from build123d import *

# Parameters (mm, degrees)
BOSS_EXTRUDE1_DEPTH = 6.35
FILLET1_R           = 6.35
SKETCH2_R           = 3.175
CUT_EXTRUDE1_DEPTH  = 6.35
BOSS_EXTRUDE2_START = 0.396875
SKETCH3_R           = 6.35
SKETCH3_R_2         = 3.175
BOSS_EXTRUDE2_DEPTH = 0.396875
SKETCH4_R           = 6.35
SKETCH4_R_2         = 3.175
BOSS_EXTRUDE3_DEPTH = 0.396875
FILLET2_R           = 1.5875
CHAMFER1_SIZE       = 3.175
FILLET3_R           = 3.175


with BuildPart() as part:
    # Sketch1 → Boss-Extrude1 (new body)
    with BuildSketch(Plane.XY):
        Polygon((0, 0), (38.1, 0), (42.964382214, -4.081701322), (59.2911875, 15.375827534), (47.023929506, 18.662829407), (35.810782514, 12.7), (0, 12.7), align=None)
    extrude(amount=BOSS_EXTRUDE1_DEPTH)

    # Fillet1
    fillet1_edges = [part.edges().sort_by_distance(p)[0] for p in [
        (47.023929506, 18.662829407, 3.175),
        (0, 0, 3.175),
        (0, 12.7, 3.175),
    ]]
    fillet(fillet1_edges, radius=FILLET1_R - 0.0001)  # a hair under: the kernel refuses the full size

    # Sketch2 → Cut-Extrude1 (cut)
    with BuildSketch(Plane.XY.offset(6.35)):
        with Locations((6.35, 6.35)):
            Circle(SKETCH2_R)
        with Locations((31.75, 6.35)):
            Circle(SKETCH2_R)
    extrude(amount=-CUT_EXTRUDE1_DEPTH, mode=Mode.SUBTRACT)

    # Sketch3 → Boss-Extrude2 (add)
    # profile 1 of 2: a face of its own
    with BuildSketch(Plane.XY.offset(6.35).offset(BOSS_EXTRUDE2_START)):
        with Locations(Location((31.75, 6.35, 0), (0, 0, 270))):
            Circle(SKETCH3_R)
        with Locations((31.75, 6.35)):
            Circle(SKETCH3_R_2, mode=Mode.SUBTRACT)
    # profile 2 of 2: a face of its own
    with BuildSketch(Plane.XY.offset(6.35).offset(BOSS_EXTRUDE2_START)):
        with Locations(Location((6.35, 6.35, 0), (0, 0, 180))):
            Circle(SKETCH3_R)
        with Locations((6.35, 6.35)):
            Circle(SKETCH3_R_2, mode=Mode.SUBTRACT)
    extrude(amount=-BOSS_EXTRUDE2_DEPTH)

    # Sketch4 → Boss-Extrude3 (add)
    # profile 1 of 2: a face of its own
    with BuildSketch(Plane(origin=(0, 0, 0), x_dir=(-1, 0, 0), z_dir=(0, 0, -1))):
        with Locations(Location((-31.75, 6.35, 0), (0, 0, 270))):
            Circle(SKETCH4_R)
        with Locations(Location((-31.75, 6.35, 0), (0, 0, 180))):
            Circle(SKETCH4_R_2, mode=Mode.SUBTRACT)
    # profile 2 of 2: a face of its own
    with BuildSketch(Plane(origin=(0, 0, 0), x_dir=(-1, 0, 0), z_dir=(0, 0, -1))):
        with Locations((-6.35, 6.35)):
            Circle(SKETCH4_R)
        with Locations(Location((-6.35, 6.35, 0), (0, 0, 180))):
            Circle(SKETCH4_R_2, mode=Mode.SUBTRACT)
    extrude(amount=BOSS_EXTRUDE3_DEPTH)

    # Fillet2
    fillet2_edges = [part.edges().sort_by_distance(p)[0] for p in [
        (59.2911875, 15.375827534, 3.175),
        (38.1, 0, 3.175),
    ]]
    fillet(fillet2_edges, radius=FILLET2_R)

    # Chamfer1
    chamfer1_edges = [part.edges().sort_by_distance(p)[0] for p in [
        (42.964382214, -4.081701322, 3.175),
    ]]
    chamfer(chamfer1_edges, length=CHAMFER1_SIZE)

    # Fillet3
    fillet3_edges = [part.edges().sort_by_distance(p)[0] for p in [
        (45.005232875, -1.649510215, 3.175),
        (40.532191107, -2.040850661, 3.175),
    ]]
    fillet(fillet3_edges, radius=FILLET3_R)


solid = part.part
Design review of the part built by this model. Coordinates are the model's own, in mm. A direction names the side the tool comes from. Coordinates: 2 decimals unless noted, no trailing zeros. Write each loop counter-clockwise with the first axis right and the second up, starting at its lowest first coordinate (ties: lowest second). Pieces come first, ordered by that corner, then holes. Notation, with made-up numbers: (83.5, 48.5) -> (92.5, 48.5) arc R23 cw to (92.5, 67.5) -> close; hole circle Ø2 at (21.25, 62). An arc over 180 degrees is marked (long way). Write each question's results on one line, items separated by ' | '. Start each with the question number.
(1) Take a section at B-B on x = 4.5. Write out the cut boundary in (y, z).
(2) Tool access review of faces 4 (the face through (21, 12.7, 3)), 5 (the face through (44.9, -1.41, 3.22)), 6 (the face through (33.657, 0.293, 6.551)): name each direction out of +Z, -Z, +X, -X, +Y, -Y from which nothing blocks a thin tool from reaching the whole face with its end or side.
(3) The part is to be moulded in two halves that separate along Y. For faces 1 (the face through (39.03, -0.78, 3.13)), 2 (the face through (19, 6, 6.35)), 3 (the face through (31.06, 9.45, 3.23)), say which applies: pulls with the +Y half, pulls with the -Y half, needs draft (parallel to the pull), parting line crosses it, or undercut.
(4) Take a section at A-A on z = 5. Give the number of separate pieces and of enclosed holes in the cut face, and give its area (3 significant figures).
(5) Take a section at C-C on y = 11. Write out the cut boundary in (x, z), and give its area (3 significant figures).
(6) Take a section at D-D on x = 30.5. Write out the cut boundary in (y, z).
(7) Clearance check with flat-ended pins moving along their axes: P1, Ø4, axis at x = 43, y = 5.5, coming from the +Z side; P2, Ø4, axis at x = 13, y = 1.5, coming from the -Z side; P3, Ø1, axis at y = 15.5, z = 2.5, coming from the -X side; P4, Ø4, axis at x = 29.5, z = 2.5, coming from the +Y side. State where each tip first meets the part, or that it passes through.
(8) For line 1 along Y through (x, z) = (31.5, 5.5); line 2 along X through (y, z) = (4, 1.75); line 3 along X through (y, z) = (6.35, 3) (3 decimals), list the stretches that pass through material, from the lowest coordinate up. Write a range as from..to.
Results found:
1) outline: (0.28, -0.4) -> (3.77, -0.4) -> (3.77, 6.75) -> (0.28, 6.75) -> (0.28, 6.35) -> close; (8.93, -0.4) -> (12.42, -0.4) -> (12.42, 6.35) -> (12.42, 6.75) -> (8.93, 6.75) -> close
2) face 4: +Z, -Z, -X, +Y | face 5: +Z, -Z, +X, -Y | face 6: +Z
3) face 1: pulls with the -Y half | face 2: needs draft | face 3: undercut
4) separate pieces: 1 | enclosed holes: 2 | area: 669 mm2
5) outline: (2.03, -0.4) -> (10.67, -0.4) -> (10.67, 0) -> (27.43, 0) -> (27.43, -0.4) -> (36.07, -0.4) -> (36.07, 0) -> (55.62, 0) -> (55.62, 6.35) -> (36.07, 6.35) -> (36.07, 6.75) -> (27.43, 6.75) -> (27.43, 6.35) -> (10.67, 6.35) -> (10.67, 6.75) -> (2.03, 6.75) -> (2.03, 6.35) -> close | area: 354 mm2
6) outline: (0, 0) -> (0.12, 0) -> (0.12, -0.4) -> (3.43, -0.4) -> (3.43, 6.75) -> (0.12, 6.75) -> (0.12, 6.35) -> (0, 6.35) -> close; (9.27, -0.4) -> (12.58, -0.4) -> (12.58, 0) -> (12.7, 0) -> (12.7, 6.35) -> (12.58, 6.35) -> (12.58, 6.75) -> (9.27, 6.75) -> close
7) P1: stops at z = 6.35 | P2: stops at z = -0.4 | P3: stops at x = 40.14 | P4: stops at y = 12.7
8) line 1: y = 0..3.18, 9.52..12.7 | line 2: x = 0.45..4.22, 8.48..29.62, 33.88..49.75 | line 3: x = 0..3.175, 9.525..28.575, 34.925..51.718
